```python
from build123d import *

# Parameters (mm, degrees)
SKETCH1_W           = 10
SKETCH1_H           = 32
BOSS_EXTRUDE1_DEPTH = 2
SKETCH2_W           = 10
SKETCH2_H           = 2
BOSS_EXTRUDE2_DEPTH = 18
SKETCH3_R           = 2.5
CUT_EXTRUDE1_DEPTH  = 2


with BuildPart() as part:
    # Sketch1 → Boss-Extrude1 (new body)
    with BuildSketch(Plane.XY):
        Rectangle(SKETCH1_W, SKETCH1_H)
    extrude(amount=BOSS_EXTRUDE1_DEPTH)

    # Sketch2 → Boss-Extrude2 (add)
    with BuildSketch(Plane.XY.offset(2)):
        with Locations((0, 15)):
            Rectangle(SKETCH2_W, SKETCH2_H)
    extrude(amount=BOSS_EXTRUDE2_DEPTH)

    # Sketch3 → Cut-Extrude1 (cut)
    with BuildSketch(Plane(origin=(0, 16, 0), x_dir=(1, 0, 0), z_dir=(0, 1, 0))):
        with Locations(Location((0, -13, 0), (0, 0, 270))):
            Circle(SKETCH3_R)
    extrude(amount=-CUT_EXTRUDE1_DEPTH, mode=Mode.SUBTRACT)


solid = part.part
```
Geometry: final body of the model. Coordinates: model frame, mm. A direction names the side the tool comes from. Coordinates: 2 decimals unless noted, no trailing zeros. Order: outer loops, then holes, each group sorted by start corner. A loop starts at its lowest first (then second) coordinate and runs counter-clockwise, first axis right, second up. Notation, with made-up numbers: (28, -2) -> (67, -2) arc R27 ccw to (67, 17) -> close; hole circle Ø11 at (-32.5, 63). An arc over 180 degrees is marked (long way). Write item = value, one per line.
(1) Access query for faces 1 (the flat face through (0, 14, 9)), 2 (the flat face through (0, 16, 10)). Directions: +Z, -Z, +X, -X, +Y, -Y. A direction counts if a zero-diameter tool reaches every point of the face in a straight line with its end or side. Return the directions, or none.
Solved:
face_1 = +Z, +X, -X, -Y
face_2 = +Z, -Z, +X, -X, +Y
(2) Cut plane B-B on z = 13. Return loops of the section in (x, y).
Solved:
outline = (-5, 14) -> (-2.5, 14) -> (-2.5, 16) -> (-5, 16) -> close; (2.5, 14) -> (5, 14) -> (5, 16) -> (2.5, 16) -> close
(3) Cut plane C-C on x = -2. Return loops of the section in (y, z), plus the area to 3 significant figures.
Solved:
outline = (-16, 0) -> (16, 0) -> (16, 11.5) -> (14, 11.5) -> (14, 2) -> (-16, 2) -> close; (14, 14.5) -> (16, 14.5) -> (16, 20) -> (14, 20) -> close
area = 94.0 mm²
(4) Pull-direction query (Z, two-part tool) for faces 3 (the cylindrical face through (0.1, 15, 10.5)), 4 (the flat face through (0, 0, 0)), 5 (the flat face through (0, 15, 20)), 6 (the flat face through (0, -16, 1)); classes: pulls with the +Z half, pulls with the -Z half, needs draft (parallel to the pull), parting line crosses it, or undercut.
Solved:
face_3 = undercut
face_4 = pulls with the -Z half
face_5 = pulls with the +Z half
face_6 = needs draft
(5) Pin query (flat end, axial travel): pin 1 Ø5 at (x, y) = (-1.5, -9.5) entering from -Z; pin 2 Ø4 at (x, y) = (3.5, -5.5) entering from +Z; pin 3 Ø1 at (x, z) = (3, 8) entering from -Y. Return the tip coordinate at first contact, or that it passes through.
Solved:
pin_1 = 0
pin_2 = 2
pin_3 = 14
(6) Cut plane D-D on y = 11.5. Return loops of the section in (x, z), plus the area to 3 significant figures.
Solved:
outline = (-5, 0) -> (5, 0) -> (5, 2) -> (-5, 2) -> close
area = 20.0 mm²
(7) Cut plane A-A on x = 0. Return loops of the section in (y, z), plus the area to 3 significant figures.
Solved:
outline = (-16, 0) -> (16, 0) -> (16, 10.5) -> (14, 10.5) -> (14, 2) -> (-16, 2) -> close; (14, 15.5) -> (16, 15.5) -> (16, 20) -> (14, 20) -> close
area = 90.0 mm²
(8) Line query: line 1 (X direction, y = 15.5, z = 13); line 2 (Y direction, x = -1.75, z = 3.5); line 3 (Z direction, x = -4.25, y = 11). Output: solid intervals per line, ascending.
Solved:
line_1 = -5 to -2.5, 2.5 to 5
line_2 = 14 to 16
line_3 = 0 to 2
